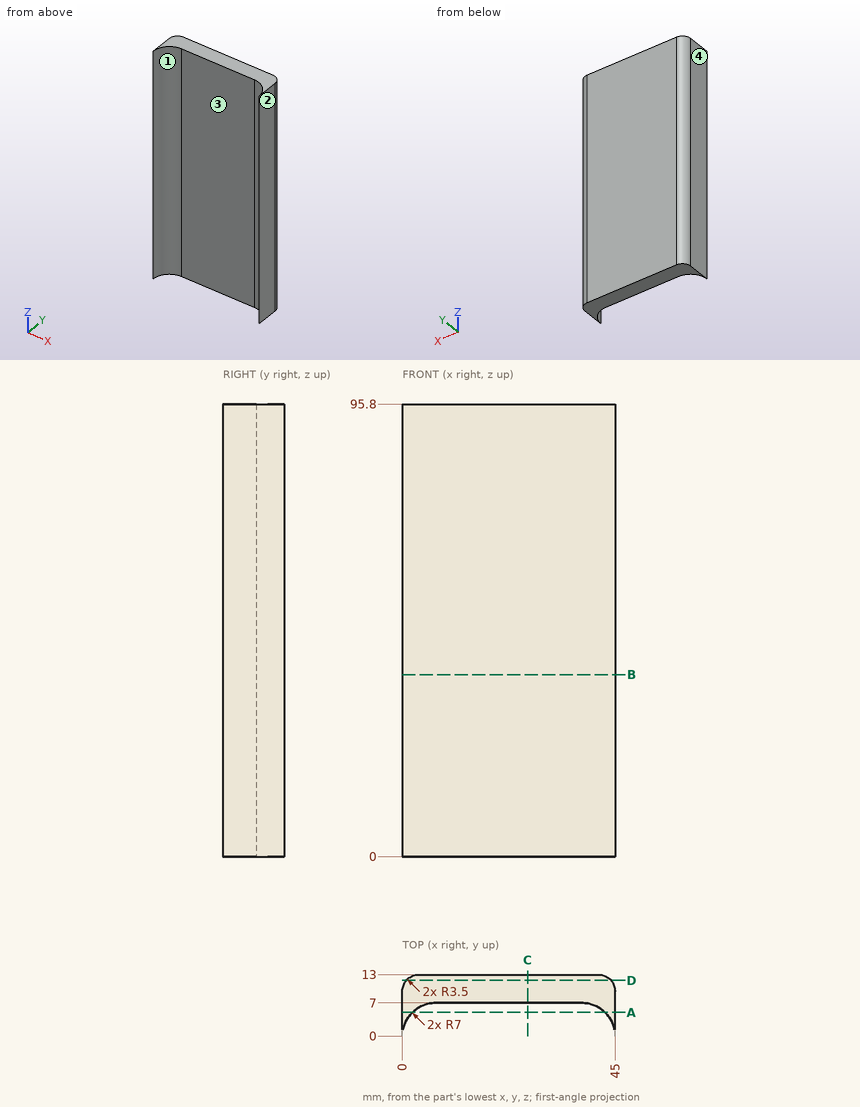
Verification items for this drawing (mm, ordinates from the low corner). Give positions to 0.01 mm unless a question says otherwise; leave off trailing zeros. Write each loop counter-clockwise with the first axis right and the second up, starting at its lowest first coordinate (ties: lowest second). Pieces come first, ordered by that corner, then holes. Notation, with made-up numbers: (4.25, 65.5) -> (51.25, 65.5) arc R28 cw to (51.25, 92.5) -> close; hole circle Ø7 at (13, -16.5). An arc over 180 degrees is marked (long way). Use CSV: the item, a comma, the result in double quotes.
(1) Release check for a two-part mould opening along X. For the marked faces 1, 2, 3 and 4 record: +X half, -X half, draft (parallel to the pull), parting line (faces both ways), or undercut.
Derived:
face 1,"undercut"
face 2,"+X half"
face 3,"undercut"
face 4,"-X half"
(2) Sectioned sample at B-B (z = 38.5). Record the cut outline in (x, y), plus the area to 3 significant figures.
Derived:
outline,"(0, 0) arc R7 cw to (7, 7) -> (38, 7) arc R7 cw to (45, 0) -> (45, 9.5) arc R3.5 ccw to (41.5, 13) -> (3.5, 13) arc R3.5 ccw to (0, 9.5) -> close"
area,"286 mm^2"
(3) Material ranges on L1, parallel to Y at x = 29, z = 54.5; L2, parallel to X at y = 6, z = 14.5; L3, parallel to Y at x = 6, z = 65, recorded low to high.
Derived:
L1,"y = 7 to 13"
L2,"x = 0 to 3.39, 41.61 to 45"
L3,"y = 6.93 to 13"
(4) Sectioned sample at C-C (x = 26.5). Record the cut outline in (y, z), plus the area to 3 significant figures.
Derived:
outline,"(7, 0) -> (13, 0) -> (13, 95.8) -> (7, 95.8) -> close"
area,"575 mm^2"
(5) Sectioned sample at D-D (y = 11.75). Record the cut outline in (x, z).
Derived:
outline,"(0.82, 0) -> (44.18, 0) -> (44.18, 95.8) -> (0.82, 95.8) -> close"
(6) Sectioned sample at A-A (y = 5). Record the cut outline in (x, z), plus the area to 3 significant figures.
Derived:
outline,"(0, 0) -> (2.1, 0) -> (2.1, 95.8) -> (0, 95.8) -> close; (42.9, 0) -> (45, 0) -> (45, 95.8) -> (42.9, 95.8) -> close"
area,"403 mm^2"
(7) Go/stop test with a flat-tipped pin: pin 1 (9.5 mm diameter, centred on x = 24.5, z = 70, fed in from -Y). Record where the tip stops, or that it passes through.
Derived:
pin 1,"stops at y = 7"
